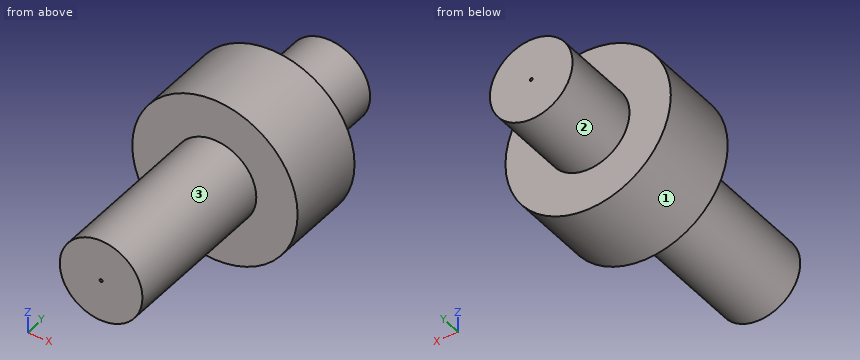
```python
from build123d import *

# Parameters (mm, degrees)
F0_R     = 63.5
F0_R_2   = 2.244615
F1_DEPTH = 508
F3_R     = 127
F4_DEPTH = 127


with BuildPart() as f1:
    # F0 (on Front) → F1 (new body)
    with BuildSketch(Plane.XZ):
        Circle(F0_R)
        Circle(F0_R_2, mode=Mode.SUBTRACT)
    extrude(amount=F1_DEPTH)

    # F3 (on offset) → F4 (join)
    with BuildSketch(Plane.XZ.offset(127)):
        Circle(F3_R)
    extrude(amount=F4_DEPTH)


solid = f1.part
```
CAD build for the part. Positions are in the model's coordinates, mm. Face numbers are marked on the shaded views. A direction names the side the tool comes from. Give positions to 0.01 mm unless a question says otherwise; leave off trailing zeros. Loops run counter-clockwise (first coordinate to the right, second up) from the corner with the lowest first, then second, coordinate; pieces in that order, holes last. Notation, with made-up numbers: (7, -33.5) - (28, -33.5) arc R23 cw to (28, 5.5) - close; hole circle Ø4 at (54, 3). An arc over 180 degrees is marked (long way). Put each result on its own line as item: value.
Q1. Slice it at B-B (z = 46.5). Give the cut face in (x, y), plus the area to 3 significant figures.
Filled in:
outline: (-118.18, -254) - (-43.24, -254) - (-43.24, -508) - (43.24, -508) - (43.24, -254) - (118.18, -254) - (118.18, -127) - (43.24, -127) - (43.24, 0) - (-43.24, 0) - (-43.24, -127) - (-118.18, -127) - close
area: 63,000 mm²
Q2. Slice it at C-C (x = 46). Give the cut face in (y, z) (3 decimals).
Filled in:
outline: (-508, -43.775) - (-254, -43.775) - (-254, -118.377) - (-127, -118.377) - (-127, -43.775) - (0, -43.775) - (0, 43.775) - (-127, 43.775) - (-127, 118.377) - (-254, 118.377) - (-254, 43.775) - (-508, 43.775) - close
Q3. Tool access for the marked faces 1, 2 and 3: list every direction of +Z, -Z, +X, -X, +Y, -Y with a clear straight run to the whole face (end or side of a thin tool).
Filled in:
face 1: +Y, -Y
face 2: +Y
face 3: -Y
Q4. Probe line 1 along X through (y, z) = (-30, 0); line 2 along Y through (x, z) = (-54.5, -113). List the from-to ranges inside material, lowest first.
Filled in:
line 1: x = -63.5 to -2.24, 2.24 to 63.5
line 2: y = -254 to -127
Q5. Slice it at A-A (y = -338). Give the cut face in (x, z).
Filled in:
outline: circle Ø127 at (0, 0); hole circle Ø4.49 at (0, 0)
Q6. Flat gauge pins, fed straight in: pin 1 (2 mm diameter, centred on x = 65.5, z = 66, fed in from -Y); pin 2 (2 mm diameter, centred on y = -71, z = 38, fed in from -X); pin 3 (10 mm diameter, centred on y = -257.5, z = -55.5, fed in from +X). Where does each tip first touch, or does it go through?
Filled in:
pin 1: stops at y = -254
pin 2: stops at x = -51.61
pin 3: stops at x = 115.9
Q7. Slice it at D-D (y = -195). Give the cut face in (x, z).
Filled in:
outline: circle Ø254 at (0, 0)
